```python
from build123d import *

# Parameters (mm, degrees)
F0_R     = 40
F1_DEPTH = 85
F2_R     = 20
F3_DEPTH = 88
F4_R     = 5
F5_R     = 33.0630902993
F5_R_2   = 20
F6_DEPTH = 6
F7_R     = 5


with BuildPart() as f1:
    # F0 (on Top) → F1 (new body)
    with BuildSketch(Plane.XY):
        Circle(F0_R)
    extrude(amount=F1_DEPTH)

    # F2 (on face) → F3 (cut)
    with BuildSketch(Plane.XY.offset(85)):
        Circle(F2_R)
    extrude(amount=-F3_DEPTH, mode=Mode.SUBTRACT)

    # F4
    f4_edges = [f1.edges().sort_by_distance(p)[0] for p in [
        (-20, 0, 0),
    ]]
    fillet(f4_edges, radius=F4_R)

    # F5 (on face) → F6 (join, symmetric)
    with BuildSketch(Plane.XY.offset(85)):
        Circle(F5_R)
        Circle(F5_R_2, mode=Mode.SUBTRACT)
    extrude(amount=F6_DEPTH, both=True)

    # F7
    f7_edges = [f1.edges().sort_by_distance(p)[0] for p in [
        (-20, 0, 79),
        (20, 0, 42),
        (-20, 0, 5),
        (-20, 0, 85),
        (20, 0, 82),
        (20, 0, 88),
        (-20, 0, 91),
    ]]
    fillet(f7_edges, radius=F7_R)


solid = f1.part
```
Design review of the part built by this model. Coordinates are the model's own, in mm. A direction names the side the tool comes from. Coordinates: 2 decimals unless noted, no trailing zeros. Order: outer loops, then holes, each group sorted by start corner. A loop starts at its lowest first (then second) coordinate and runs counter-clockwise, first axis right, second up. Notation, with made-up numbers: (7.25, 30) -> (35.25, 30) arc R24 cw to (35.25, 48) -> close; hole circle Ø9 at (64, 24.5). An arc over 180 degrees is marked (long way). One line per item, written item: value. Start each with the question number.
Q1. Mouldability with a two-part tool opening along X and no side actions: class faces 1 (the cylindrical face through (-8.67, -39.05, 41.9)), 2 (the cylindrical face through (-4.336, -19.524, 46.067)), 3 (the flat face through (-15, 30, 85)) as pulls with the +X half, pulls with the -X half, needs draft (parallel to the pull), parting line crosses it, or undercut.
Q2. Take a section at C-C, the plane z = 52.5. State the section outline as (x, y) points, then the cut area to 3 significant figures.
Q3. Take a section at A-A, the plane x = 0. State the section outline as (y, z) points.
Q4. For probe 1 along Y at (x, z) = (0, 48); probe 2 along X at (y, z) = (-17.5, 50); probe 3 along Y at (x, z) = (10.5, 61.5), list the stretches that pass through material, from the lowest coordinate up.
Q5. Insertion check: pin 1 Ø10 at (y, z) = (-7.5, 66.5) entering from -X; pin 2 Ø1 at (y, z) = (2, 13) entering from -X; pin 3 Ø2 at (x, y) = (-19.5, -2) entering from -Z; pin 4 Ø3 at (x, y) = (14, -11.5) entering from +Z. Each pin has a flat end and moves straight along its axis. Give the tip position at first contact, or say it passes through.
Q6. Tool access review of faces 4 (the flat face through (17.22, 18.34, 0)), 5 (the cylindrical face through (30.542, -12.663, 88.042)): name each direction out of +Z, -Z, +X, -X, +Y, -Y from which nothing blocks a thin tool from reaching the whole face with its end or side.
Q7. Take a section at D-D, the plane x = -28.5. State the section outline as (y, z) points, then the cut area to 3 significant figures.
Values follow:
1. face 1: parting line crosses it
1. face 2: undercut
1. face 3: needs draft
2. outline: circle Ø80 at (0, 0); hole circle Ø40 at (0, 0)
2. area: 3,770 mm2
3. outline: (-40, 0) -> (-25, 0) arc R5 ccw to (-20, 5) -> (-20, 86) arc R5 ccw to (-25, 91) -> (-33.06, 91) -> (-33.06, 85) -> (-40, 85) -> close; (20, 5) arc R5 ccw to (25, 0) -> (40, 0) -> (40, 85) -> (33.06, 85) -> (33.06, 91) -> (25, 91) arc R5 ccw to (20, 86) -> close
4. probe 1: y = -40 to -20, 20 to 40
4. probe 2: x = -35.97 to -9.68, 9.68 to 35.97
4. probe 3: y = -38.6 to -17.02, 17.02 to 38.6
5. pin 1: stops at x = -39.92
5. pin 2: stops at x = -39.97
5. pin 3: stops at z = 2.62
5. pin 4: passes through
6. face 4: -Z, +X, -X, +Y, -Y
6. face 5: +Z
7. outline: (-28.07, 0) -> (28.07, 0) -> (28.07, 85) -> (16.76, 85) -> (16.76, 91) -> (-16.76, 91) -> (-16.76, 85) -> (-28.07, 85) -> close
7. area: 4,970 mm2
